from build123d import *

# Parameters (mm, degrees)
SKETCH_1_W                  = 55
SKETCH_1_H                  = 75
EXTRUDE_1_DEPTH             = 14
SKETCH_2_W                  = 50
SKETCH_2_H                  = 70
CUT_EXTRUDE_1_DEPTH         = 6
SKETCH_3_W                  = 17
SKETCH_3_H                  = 21
SKETCH_3_H_2                = 16
SKETCH_3_W_2                = 8
CUT_EXTRUDE_2_DEPTH         = 12
CUT_EXTRUDE_3_REACH         = 50.026
PATTERN_LINEAR_1_COUNT      = 2
PATTERN_LINEAR_1_PITCH      = 34
PATTERN_LINEAR_1_COUNT_DIR2 = 2
PATTERN_LINEAR_1_PITCH_DIR2 = 20
CHAMFER_1_SIZE              = 3


with BuildPart() as part:
    # 草图1 → 凸台-拉伸1 (new body)
    with BuildSketch(Plane(origin=(0, 0, 0), x_dir=(1, 0, 0), z_dir=(0, 1, 0))):
        Rectangle(SKETCH_1_W, SKETCH_1_H)
    extrude(amount=EXTRUDE_1_DEPTH)

    # 草图2 → 切除-拉伸1 (cut)
    with BuildSketch(Plane(origin=(0, 14, 0), x_dir=(1, 0, 0), z_dir=(0, 1, 0))):
        with Locations((-2.5, 2.5)):
            Rectangle(SKETCH_2_W, SKETCH_2_H)
    extrude(amount=-CUT_EXTRUDE_1_DEPTH, mode=Mode.SUBTRACT)

    # 草图3 → 切除-拉伸2 (cut)
    with BuildSketch(Plane(origin=(0, 14, 0), x_dir=(1, 0, 0), z_dir=(0, 1, 0))):
        with Locations((19, -27)):
            Rectangle(SKETCH_3_W, SKETCH_3_H)
        with Locations((19, 29.5)):
            Rectangle(SKETCH_3_W, SKETCH_3_H_2)
        with Locations((-23.5, 29.5)):
            Rectangle(SKETCH_3_W_2, SKETCH_3_H_2)
        with Locations((-23.5, -27)):
            Rectangle(SKETCH_3_W_2, SKETCH_3_H)
    extrude(amount=-CUT_EXTRUDE_2_DEPTH, mode=Mode.SUBTRACT)

    # 草图4 → 切除-拉伸3 (cut, up to next)
    with BuildSketch(Plane(origin=(0, 2, 0), x_dir=(1, 0, 0), z_dir=(0, 1, 0)), mode=Mode.PRIVATE) as cut_extrude_3_sk1:
        with BuildLine():
            Line((-21.25, 32.25), (-21.25, 26.75))
            ThreePointArc((-21.25, 26.75), (-23.5, 24.5), (-25.75, 26.75))
            Line((-25.75, 26.75), (-25.75, 32.25))
            ThreePointArc((-25.75, 32.25), (-23.5, 34.5), (-21.25, 32.25))
        make_face()
    cut_extrude_3_tool1 = extrude(cut_extrude_3_sk1.sketch, amount=-CUT_EXTRUDE_3_REACH, mode=Mode.PRIVATE) & part.part
    # 草图4 → 切除-拉伸3 (cut, up to next)
    with BuildSketch(Plane(origin=(0, 2, 0), x_dir=(1, 0, 0), z_dir=(0, 1, 0)), mode=Mode.PRIVATE) as cut_extrude_3_sk2:
        with BuildLine():
            Line((16.75, 32.25), (16.75, 26.75))
            ThreePointArc((16.75, 26.75), (14.5, 24.5), (12.25, 26.75))
            Line((12.25, 26.75), (12.25, 32.25))
            ThreePointArc((12.25, 32.25), (14.5, 34.5), (16.75, 32.25))
        make_face()
    cut_extrude_3_tool2 = extrude(cut_extrude_3_sk2.sketch, amount=-CUT_EXTRUDE_3_REACH, mode=Mode.PRIVATE) & part.part
    # 草图4 → 切除-拉伸3 (cut, up to next)
    with BuildSketch(Plane(origin=(0, 2, 0), x_dir=(1, 0, 0), z_dir=(0, 1, 0)), mode=Mode.PRIVATE) as cut_extrude_3_sk3:
        with BuildLine():
            Line((16.75, -21.75), (16.75, -27.25))
            ThreePointArc((16.75, -27.25), (14.5, -29.5), (12.25, -27.25))
            Line((12.25, -27.25), (12.25, -21.75))
            ThreePointArc((12.25, -21.75), (14.5, -19.5), (16.75, -21.75))
        make_face()
    cut_extrude_3_tool3 = extrude(cut_extrude_3_sk3.sketch, amount=-CUT_EXTRUDE_3_REACH, mode=Mode.PRIVATE) & part.part
    # 草图4 → 切除-拉伸3 (cut, up to next)
    with BuildSketch(Plane(origin=(0, 2, 0), x_dir=(1, 0, 0), z_dir=(0, 1, 0)), mode=Mode.PRIVATE) as cut_extrude_3_sk4:
        with BuildLine():
            Line((-21.25, -21.75), (-21.25, -27.25))
            ThreePointArc((-21.25, -27.25), (-23.5, -29.5), (-25.75, -27.25))
            Line((-25.75, -27.25), (-25.75, -21.75))
            ThreePointArc((-25.75, -21.75), (-23.5, -19.5), (-21.25, -21.75))
        make_face()
    cut_extrude_3_tool4 = extrude(cut_extrude_3_sk4.sketch, amount=-CUT_EXTRUDE_3_REACH, mode=Mode.PRIVATE) & part.part
    add(cut_extrude_3_tool1.solids().sort_by_distance((-23.5, 2, -29.5))[0], mode=Mode.SUBTRACT)
    add(cut_extrude_3_tool2.solids().sort_by_distance((14.5, 2, -29.5))[0], mode=Mode.SUBTRACT)
    add(cut_extrude_3_tool3.solids().sort_by_distance((14.5, 2, 24.5))[0], mode=Mode.SUBTRACT)
    add(cut_extrude_3_tool4.solids().sort_by_distance((-23.5, 2, 24.5))[0], mode=Mode.SUBTRACT)

    # 草图7 → M4 螺纹孔1 (revolve, cut)
    with BuildSketch(Plane(origin=(-21.5, 8, -12.5), x_dir=(0, 0, 1), z_dir=(1, 0, 0))):
        Polygon((0, 0), (0, 11.091420021), (1.65, 10.1), (1.65, 0), align=None)
    hole_wizard_m4_1 = revolve(axis=Axis((-21.5, 14.35, -12.5), (0, -1, 0)), mode=Mode.SUBTRACT)

    # 阵列(线性)1: Hole Wizard M4 _1 2 × 2
    with Locations(*[(i * PATTERN_LINEAR_1_PITCH, 0, j * PATTERN_LINEAR_1_PITCH_DIR2) for i in range(PATTERN_LINEAR_1_COUNT) for j in range(PATTERN_LINEAR_1_COUNT_DIR2) if (i, j) != (0, 0)]):
        add(hole_wizard_m4_1, mode=Mode.SUBTRACT)

    # 倒角1
    chamfer_1_edges = [part.edges().sort_by_distance(p)[0] for p in [
        (27.5, 1, -37.5),
        (-27.5, 1, -37.5),
        (27.5, 1, 37.5),
        (-27.5, 1, 37.5),
    ]]
    chamfer(chamfer_1_edges, length=CHAMFER_1_SIZE)


solid = part.part
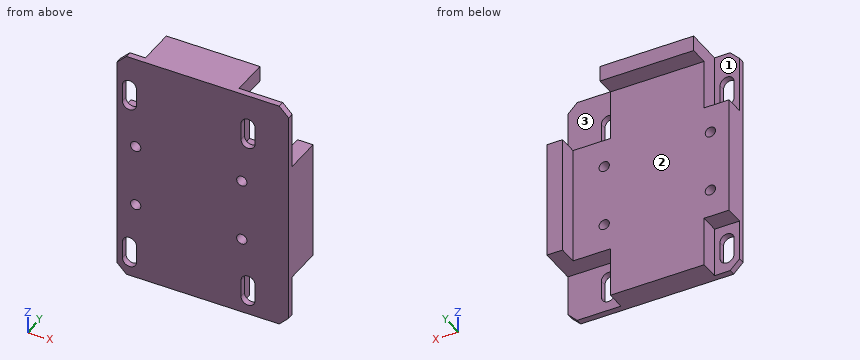
Part model, mm, in its own coordinate system. Face numbers are marked on the shaded views. A direction names the side the tool comes from. Round coordinates to 2 decimals unless told otherwise and drop trailing zeros. Loops run counter-clockwise (first coordinate to the right, second up) from the corner with the lowest first, then second, coordinate; pieces in that order, holes last. Notation, with made-up numbers: (34, -20.75) - (49, -20.75) arc R6 cw to (49, -10.75) - close; hole circle Ø7 at (50.5, -15.75). An arc over 180 degrees is marked (long way). Answer as a JSON object with one key per item and string values.
Item 1: Band-saw the part on D-D on x = 2.5. List the corners of the cut face in (y, z).
Output:
{"outline": "(0, -37.5) - (8, -37.5) - (8, 32.5) - (14, 32.5) - (14, 37.5) - (0, 37.5) - close"}
Item 2: Pin check, flat tips, straight feed: pin 1 (5 mm diameter, centred on y = 5.5, z = 25.5, fed in from -X); pin 2 (5 mm diameter, centred on y = 5.5, z = -27, fed in from +X); pin 3 (6.5 mm diameter, centred on y = 12, z = -3.5, fed in from -X); pin 4 (2.5 mm diameter, centred on x = 12.5, z = 7.5, fed in from +Y). Stop position of each tip, or through.
Output:
{"pin 1": "x = -19.5", "pin 2": "x = 10.5", "pin 3": "x = 22.5", "pin 4": "through"}
Item 3: Band-saw the part on A-A on z = 7.5. List the corners of the cut face in (x, y), plus the area to 3 significant figures.
Output:
{"outline": "(-27.5, 0) - (-23.15, 0) - (-23.15, 8) - (-27.5, 8) - close; (-19.85, 0) - (10.85, 0) - (10.85, 8) - (-19.85, 8) - close; (14.15, 0) - (27.5, 0) - (27.5, 14) - (22.5, 14) - (22.5, 8) - (14.15, 8) - close", "area": "417 mm2"}
Item 4: Band-saw the part on C-C on z = 25. List the corners of the cut face in (x, y).
Output:
{"outline": "(-27.5, 0) - (-25.75, 0) - (-25.75, 2) - (-27.5, 2) - close; (-21.25, 0) - (12.25, 0) - (12.25, 2) - (10.5, 2) - (10.5, 8) - (-19.5, 8) - (-19.5, 2) - (-21.25, 2) - close; (16.75, 0) - (27.5, 0) - (27.5, 2) - (16.75, 2) - close"}
Item 5: Wall check: L1, parallel to X at y = 4, z = -12.5; L2, parallel to Z at x = 12.5, y = 4.5; L3, parallel to X at y = 1, z = 26.5. Give the ranges that are in metal, low to high.
Output:
{"L1": "-27.5 to -23.15, -19.85 to 10.85, 14.15 to 27.5", "L2": "-21.5 to -14.15, -10.85 to 5.85, 9.15 to 16.5", "L3": "-27.5 to -25.75, -21.25 to 12.25, 16.75 to 27.5"}
Item 6: Band-saw the part on B-B on y = 3.25. List the corners of the cut face in (x, z), plus the area to 3 significant figures.
Output:
{"outline": "(-27.5, -21.5) - (-19.5, -21.5) - (-19.5, -37.5) - (10.5, -37.5) - (10.5, -21.5) - (27.5, -21.5) - (27.5, 16.5) - (10.5, 16.5) - (10.5, 37.5) - (-19.5, 37.5) - (-19.5, 16.5) - (-27.5, 16.5) - close; hole circle Ø3.3 at (-21.5, -12.5); hole circle Ø3.3 at (-21.5, 7.5); hole circle Ø3.3 at (12.5, -12.5); hole circle Ø3.3 at (12.5, 7.5)", "area": "3,170 mm2"}
Item 7: Tool access for the marked faces 1, 2 and 3: list every direction of +Z, -Z, +X, -X, +Y, -Y with a clear straight run to the whole face (end or side of a thin tool).
Output:
{"face 1": "+Z, -X, +Y", "face 2": "-Z, -X, +Y", "face 3": "+Z, +X, +Y"}
